Design review of the part built by this model. Coordinates are the model's own, in mm. A direction names the side the tool comes from. Round coordinates to 2 decimals unless told otherwise and drop trailing zeros. Loops run counter-clockwise (first coordinate to the right, second up) from the corner with the lowest first, then second, coordinate; pieces in that order, holes last. Notation, with made-up numbers: (71, -6.5) - (111, -6.5) arc R12 cw to (111, 13.5) - close; hole circle Ø1 at (-14.75, 22). An arc over 180 degrees is marked (long way). Return JSON: item names as keys, results as strings. Group by question number.
from build123d import *

# Parameters (mm, degrees)
SKETCH_2_W            = 27
SKETCH_2_H            = 15
EXTRUDE_1_DEPTH       = 22.2
SHELL_2_T             = -4
SKETCH_3_R            = 1
CUT_EXTRUDE_1_DEPTH   = 32.2
SKETCH_4_W            = 50
SKETCH_4_H            = 15
EXTRUDE_2_DEPTH       = 4
SKETCH_5_W            = 19
SKETCH_5_H            = 15
CUT_EXTRUDE_2_DEPTH   = 8
F_3_0MM_1_D           = 3
F_3_0MM_1_CSINK_D     = 3.05
F_3_0MM_1_CSINK_ANGLE = 90


with BuildPart() as part:
    # Sketch 2 → Extrude 1 (new body)
    with BuildSketch(Plane(origin=(0, 0, 0), x_dir=(1, 0, 0), z_dir=(0, 1, 0))):
        with Locations((13.5, 7.5)):
            Rectangle(SKETCH_2_W, SKETCH_2_H)
    extrude(amount=EXTRUDE_1_DEPTH)

    # Shell 2
    shell_2_openings = [part.faces().sort_by_distance(p)[0] for p in [
        (13.5, 22.2, -7.5),
        (13.5, 11.1, -15),
        (13.5, 11.1, 0),
    ]]
    offset(amount=SHELL_2_T, openings=shell_2_openings, kind=Kind.INTERSECTION)

    # Sketch 3 → Cut-Extrude 1 (cut)
    with BuildSketch(Plane.ZY):
        with Locations((-15, 11.1)):
            Circle(SKETCH_3_R)
    extrude(amount=-CUT_EXTRUDE_1_DEPTH, mode=Mode.SUBTRACT)

    # Sketch 4 → Extrude 2 (add)
    with BuildSketch(Plane(origin=(0, 22.2, 0), x_dir=(1, 0, 0), z_dir=(0, 1, 0))):
        with Locations((13.5, 7.5)):
            Rectangle(SKETCH_4_W, SKETCH_4_H)
    extrude(amount=EXTRUDE_2_DEPTH)

    # Sketch 5 → Cut-Extrude 2 (cut)
    with BuildSketch(Plane.XZ.offset(-22.2)):
        with Locations((13.5, -7.5)):
            Rectangle(SKETCH_5_W, SKETCH_5_H)
    extrude(amount=-CUT_EXTRUDE_2_DEPTH, mode=Mode.SUBTRACT)

    # 3.0mm _1 (through all)
    with Locations(Plane(origin=(0, 26.2, 0), x_dir=(1, 0, 0), z_dir=(0, 1, 0))):
        with Locations((-3.5, 11.5), (-3.5, 3.5), (30.5, 11.5), (30.5, 3.5)):
            CounterSinkHole(F_3_0MM_1_D / 2, F_3_0MM_1_CSINK_D / 2, counter_sink_angle=F_3_0MM_1_CSINK_ANGLE)


solid = part.part
Q1. Add section A-A, the plane z = -3.5. State the section outline as (x, y) points (3 decimals), plus the area to 3 significant figures.
Q2. Insertion check: pin 1 Ø2.5 at (x, z) = (30.5, -3.5) entering from +Y; pin 2 Ø6 at (x, z) = (-7.5, -11) entering from -Y; pin 3 Ø8 at (x, z) = (17, -12) entering from +Y. Each pin has a flat end and moves straight along its axis. Give the tip position at first contact, or say it passes through.
Q3. Add section D-D, the plane z = -13.5. State the section outline as (x, y) points.
Q4. Add section B-B, the plane y = 11.1. State the section outline as (x, z) points.
Q5. Add section C-C, the plane x = 30.5. State the section outline as (y, z) points (3 decimals), plus the area to 3 significant figures.
Q6. For line 1 (Z direction, x = -3.5, y = 23.1); line 2 (X direction, y = 7.25, z = -1); line 3 (X direction, y = 23.4, z = -11.5), list the stretches that pass through material, from the lowest coordinate up.
Q7. Tool access review of faces 1 (the cylindrical face through (2, 11.1, -14)), 2 (the flat face through (27, 11, -7)), 3 (the flat face through (4, 15, -7)), 4 (the flat face through (-6, 22.2, -8)): name each direction out of +Z, -Z, +X, -X, +Y, -Y from which nothing blocks a thin tool from reaching the whole face with its end or side.
Q8. Draft analysis for pull direction Z (two halves, no side actions). For faces 5 (the cylindrical face through (32, 24.16, -11.57)), 6 (the flat face through (13, 4, -8)), 7 (the cylindrical face through (-4.886, 24.16, -2.925)), 8 (the cylindrical face through (25, 11.1, -14)), state which applies: pulls with the +Z half, pulls with the -Z half, needs draft (parallel to the pull), parting line crosses it, or undercut.
Evaluation:
{
 "1": {"outline": "(-11.5, 22.2) - (-5, 22.2) - (-5, 26.175) - (-5.025, 26.2) - (-11.5, 26.2) - close; (-2, 22.2) - (0, 22.2) - (0, 0) - (27, 0) - (27, 22.2) - (29, 22.2) - (29, 26.175) - (28.975, 26.2) - (23, 26.2) - (23, 4) - (4, 4) - (4, 26.2) - (-1.975, 26.2) - (-2, 26.175) - close; (32, 22.2) - (38.5, 22.2) - (38.5, 26.2) - (32.025, 26.2) - (32, 26.175) - close", "area": "354 mm²"},
 "2": {"pin 1": "through", "pin 2": "y = 22.2", "pin 3": "y = 4"},
 "3": {"outline": "(-11.5, 22.2) - (0, 22.2) - (0, 0) - (27, 0) - (27, 22.2) - (38.5, 22.2) - (38.5, 26.2) - (23, 26.2) - (23, 4) - (4, 4) - (4, 26.2) - (-11.5, 26.2) - close"},
 "4": {"outline": "(0, -14) - (4, -14) - (4, 0) - (0, 0) - close; (23, -14) - (27, -14) - (27, 0) - (23, 0) - close"},
 "5": {"outline": "(22.2, -15) - (26.2, -15) - (26.2, -13.025) - (26.175, -13) - (22.2, -13) - close; (22.2, -10) - (26.175, -10) - (26.2, -9.975) - (26.2, -5.025) - (26.175, -5) - (22.2, -5) - close; (22.2, -2) - (26.175, -2) - (26.2, -1.975) - (26.2, 0) - (22.2, 0) - close", "area": "36.0 mm²"},
 "6": {"line 1": "-15 to -13, -10 to -5, -2 to 0", "line 2": "0 to 4, 23 to 27", "line 3": "-11.5 to -5, -2 to 4, 23 to 29, 32 to 38.5"},
 "7": {"face 1": "-Z, +X, -X", "face 2": "+Z, -Z, +X, -Y", "face 3": "+Z, -Z, +Y", "face 4": "+Z, -Z, -X, -Y"},
 "8": {"face 5": "undercut", "face 6": "needs draft", "face 7": "undercut", "face 8": "pulls with the -Z half"}
}
